from build123d import *

# Parameters (mm, degrees)
F0_W     = 840
F0_H     = 250
F0_W_2   = 250
F0_H_2   = 150
F1_DEPTH = 10
F3_DEPTH = 100
F5_DEPTH = 10


with BuildPart() as f1:
    # F0 (on Front) → F1 (new body)
    with BuildSketch(Plane.XZ):
        Rectangle(F0_W, F0_H)
        Rectangle(F0_W_2, F0_H_2, mode=Mode.SUBTRACT)
    extrude(amount=F1_DEPTH)

    # F2 (on face) → F3 (join)
    with BuildSketch(Plane(origin=(0, 0, 0), x_dir=(-1, 0, 0), z_dir=(0, 1, 0))):
        Polygon((350, -115), (350, -125), (420, -125), (420, 73.963337), (410, 73.963337), (410, -115), align=None)
        Polygon((-410, -115), (-410, 73.963337), (-420, 73.963337), (-420, -125), (-350, -125), (-350, -115), align=None)
    extrude(amount=F3_DEPTH)

    # F4 (on face) → F5 (join)
    with BuildSketch(Plane.YZ.offset(420)):
        Polygon((228.108257, 0), (100, 73.963337), (100, -125), (228.108257, -198.963337), align=None)
        Polygon((378.108257, 0), (228.108257, 0), (228.108257, -198.963337), (378.108257, -198.963331), align=None)
    extrude(amount=-F5_DEPTH)


solid = f1.part
Can you work these out from the model? Positions are in its coordinate system, mm. A direction names the side the tool comes from. Give positions to 0.01 mm unless a question says otherwise; leave off trailing zeros. Order: outer loops, then holes, each group sorted by start corner. A loop starts at its lowest first (then second) coordinate and runs counter-clockwise, first axis right, second up. Notation, with made-up numbers: M -8,19.5 L 30,19.5 A20 cw 30,55.5 Z; hole C 12,-18 d1. An arc over 180 degrees is marked long. Use one line per item in the form item = value. Start each with the question number.
Item 1: We'd pull the mould along X, two halves only. Please class faces 1 (the flat face through (420, 181, -71)), 2 (the flat face through (380, 49, -115)), 3 (the flat face through (415.07, 164.951, 36.464)): +X half, -X half, draft (parallel to the pull), parting line (faces both ways), or undercut.
Item 2: If I drill on line 1 along X through (y, z) = (54, -113); line 2 along Z through (x, y) = (371, 53); line 3 along X through (y, z) = (117.5, -129.5), over which ranges is the centre line in solid material (lowest first)?
Item 3: If we section it at A-A (z = -65.5): Write out the boundary of the cut face in (x, y).
Item 4: Will these pins go through, and if not, where does the flat tip stop? pin 1 Ø21 at (x, z) = (-389, -11) entering from +Y; pin 2 Ø3 at (x, z) = (385.5, -120) entering from +Y; pin 3 Ø3 at (x, y) = (-414.5, 49.5) entering from +Z.
Item 5: If we section it at B-B (y = 14.5): Write out the boundary of the cut face in (x, z).
Item 6: For faces 4 (the flat face through (-410, 49, -19)), 5 (the flat face through (-413, 100, -40)), 6 (the flat face through (-6, -10, 85)), which set-ups out of +Z, -Z, +X, -X, +Y, -Y let a thin tool reach every point of the face, with its end or its side?
Item 7: If we section it at D-D (y = 248): Write out the boundary of the cut face in (x, z), then the cut area to 3 significant figures.
Item 8: If we section it at C-C (x = 37): Write out the boundary of the cut face in (y, z), then the cut area to 3 significant figures.
Outcome:
q1.face_1 = +X half
q1.face_2 = undercut
q1.face_3 = draft
q2.line_1 = -420 to -410, 410 to 420
q2.line_2 = -125 to -115
q2.line_3 = 410 to 420
q3.outline = M -420,-10 L -125,-10 L -125,0 L -410,0 L -410,100 L -420,100 Z; M 125,-10 L 420,-10 L 420,378.11 L 410,378.11 L 410,0 L 125,0 Z
q4.pin_1 = 0
q4.pin_2 = 100
q4.pin_3 = 73.96
q5.outline = M -420,-125 L -350,-125 L -350,-115 L -410,-115 L -410,73.96 L -420,73.96 Z; M 350,-125 L 420,-125 L 420,73.96 L 410,73.96 L 410,-115 L 350,-115 Z
q6.face_4 = +Z, +Y
q6.face_5 = +Z, -Z, -X, +Y
q6.face_6 = +Z, -Z, +X, -X, -Y
q7.outline = M 410,-198.96 L 420,-198.96 L 420,0 L 410,0 Z
q7.area = 1,990 mm2
q8.outline = M -10,-125 L 0,-125 L 0,-75 L -10,-75 Z; M -10,75 L 0,75 L 0,125 L -10,125 Z
q8.area = 1,000 mm2
